Work out the finished part from the listing and answer in its coordinate system (mm). A direction names the side the tool comes from. Coordinates: 2 decimals unless noted, no trailing zeros. Order: outer loops, then holes, each group sorted by start corner. A loop starts at its lowest first (then second) coordinate and runs counter-clockwise, first axis right, second up.
1. Find the intervals of material crossed by probe 1 along X at (y, z) = (-66, 225); probe 2 along Z at (x, y) = (164.5, -184), in increasing order.
2. The part is cut by section B-B, the plane x = 113.5. Give the vertices of the cut face in (y, z).
3. The part is cut by section D-D, the plane y = -130. Give the vertices of the cut face in (x, z).
4. Determine the mould class of faces 1 (the flat face through (148, -104, 20)), 2 (the flat face through (109.089, -126, 321)), 3 (the flat face through (148, -123, 0)), 4 (the flat face through (148, -84, 360)) for opening direction Z: +Z half, -Z half, draft (parallel to the pull), parting line (faces both ways), or undercut.
5. A tool of negligible diameter and unlimited length cuts with its end or side. For faces 5 (the flat face through (20, -104, 152)), 6 (the flat face through (89.089, -126, 330)), 7 (the flat face through (189.089, -126, 321)), 8 (the flat face through (148, -65, 330)), 9 (the flat face through (209.089, -126, 330)), from which of +Z, -Z, +X, -X, +Y, -Y can it reach the whole face along a straight path? Write none if from no direction.
6. The part is cut by section C-C, the plane z = 77. Give the vertices of the cut face in (x, y), then the cut area to 3 significant figures.
7. The part is cut by section A-A, the plane y = -24. Give the vertices of the cut face in (x, z).
8. Flat-ended cylindrical pins translate along their axes: pin 1 Ø4 at (x, y) = (32.5, -212) entering from -Z; pin 2 Ø6 at (x, y) = (46.5, -155.5) entering from +Z. Find the tip coordinate at first contact, or state that the pin passes through.
```python
from build123d import *

# Parameters (mm, degrees)
SKETCH2_W           = 300
SKETCH2_H           = 300
BOSS_EXTRUDE1_DEPTH = 250
SKETCH4_W           = 260
SKETCH4_H           = 260
CUT_EXTRUDE2_DEPTH  = 210
SKETCH6_W           = 120
SKETCH6_H           = 120
BOSS_EXTRUDE2_DEPTH = 60
CUT_EXTRUDE7_REACH  = 362
SKETCH11_W          = 80
SKETCH11_H          = 80


with BuildPart() as part:
    # Sketch2 → Boss-Extrude1 (new body)
    with BuildSketch(Plane(origin=(0, 0, 0), x_dir=(1, 0, 0), z_dir=(0, 1, 0))):
        with Locations((150, -150)):
            Rectangle(SKETCH2_W, SKETCH2_H)
    extrude(amount=-BOSS_EXTRUDE1_DEPTH)

    # Sketch4 → Cut-Extrude2 (cut)
    with BuildSketch(Plane(origin=(0, 0, 0), x_dir=(1, 0, 0), z_dir=(0, 1, 0))):
        with Locations((150, -150)):
            Rectangle(SKETCH4_W, SKETCH4_H)
    extrude(amount=-CUT_EXTRUDE2_DEPTH, mode=Mode.SUBTRACT)

    # Sketch6 → Boss-Extrude2 (add)
    with BuildSketch(Plane.XY.offset(300)):
        with Locations((149.088747211, -125)):
            Rectangle(SKETCH6_W, SKETCH6_H)
    extrude(amount=BOSS_EXTRUDE2_DEPTH)

    # Sketch11 → Cut-Extrude7 (cut, up to next)
    with BuildSketch(Plane.XY.offset(360), mode=Mode.PRIVATE) as cut_extrude7_sk1:
        with Locations((149.088747211, -125)):
            Rectangle(SKETCH11_W, SKETCH11_H)
    cut_extrude7_tool1 = extrude(cut_extrude7_sk1.sketch, amount=-CUT_EXTRUDE7_REACH, mode=Mode.PRIVATE) & part.part
    add(cut_extrude7_tool1.solids().sort_by_distance((149.088747, -125, 360))[0], mode=Mode.SUBTRACT)


solid = part.part
```
Geometry says:
1. probe 1: x = 0 to 20, 280 to 300
1. probe 2: z = 0 to 20, 280 to 360
2. outline: (-250, 0) - (0, 0) - (0, 20) - (-210, 20) - (-210, 280) - (-165, 280) - (-165, 360) - (-185, 360) - (-185, 300) - (-250, 300) - close; (-85, 280) - (0, 280) - (0, 300) - (-65, 300) - (-65, 360) - (-85, 360) - close
3. outline: (0, 0) - (300, 0) - (300, 300) - (209.09, 300) - (209.09, 360) - (189.09, 360) - (189.09, 280) - (280, 280) - (280, 20) - (20, 20) - (20, 280) - (109.09, 280) - (109.09, 360) - (89.09, 360) - (89.09, 300) - (0, 300) - close
4. face 1: undercut
4. face 2: draft
4. face 3: -Z half
4. face 4: +Z half
5. face 5: +Y
5. face 6: +Z, -X, +Y, -Y
5. face 7: +Z
5. face 8: +Z, +X, -X, +Y
5. face 9: +Z, +X, +Y, -Y
6. outline: (0, -250) - (300, -250) - (300, 0) - (280, 0) - (280, -210) - (20, -210) - (20, 0) - (0, 0) - close
6. area: 20,400 mm2
7. outline: (0, 0) - (300, 0) - (300, 300) - (0, 300) - close; hole (20, 20) - (280, 20) - (280, 280) - (20, 280) - close
8. pin 1: stops at z = 0
8. pin 2: stops at z = 300
